Geometry: final body of the model. Coordinates: model frame, mm. A direction names the side the tool comes from. Give positions to 0.01 mm unless a question says otherwise; leave off trailing zeros. Write each loop counter-clockwise with the first axis right and the second up, starting at its lowest first coordinate (ties: lowest second). Pieces come first, ordered by that corner, then holes.
Q1. Reachability of faces 1 (the flat face through (-13, -8, 31)), 2 (the cylindrical face through (74.856, -19.944, -1.724)), 3 (the flat face through (-12, -16, 31)), 4 (the flat face through (35.699, -12, 17)) from +Z, -Z, +X, -X, +Y, -Y: full face, straight path, thin tool, end or side. Return the list, or none.
Q2. Section B-B (y = -4.75). Return the cut outline in (x, z).
Q3. Pin query (flat end, axial travel): pin 1 Ø1 at (y, z) = (-3.5, 25.5) entering from -X; pin 2 Ø1.5 at (x, y) = (53.5, -8.5) entering from +Z; pin 3 Ø2 at (x, y) = (33, -12.5) entering from +Z; pin 4 Ø14.5 at (x, z) = (46.7, 0) entering from -Y. Return the tip coordinate at first contact, or that it passes through.
Q4. Mould query, pull axis X, two halves, no side actions, for faces 5 (the flat face through (53, -8, 11)), 6 (the cylindrical face through (50.992, -19.944, 1.352)), 7 (the cylindrical face through (44.71, -17.17, 28.79)). Classes: +X half, -X half, draft (parallel to the pull), parting line (faces both ways), or undercut.
Q5. Line query: line 1 (Y direction, x = 48, z = 7); line 2 (Z direction, x = 45, y = -4.5); line 3 (X direction, y = -18.5, z = 3.5). Output: solid intervals per line, ascending.
Q6. Section A-A (x = 61.5). Return the cut outline in (y, z), plus the area to 3 significant figures.
Q7. Section D-D (y = -22). Return the cut outline in (x, z), plus the area to 3 significant figures.
Q8. Section C-C (z = 7.5). Return the cut outline in (x, y), plus the area to 3 significant figures.
from build123d import *

# Parameters (mm, degrees)
F0_R          = 4.5
F1_DEPTH      = 24
F2_W          = 44
F2_H          = 8
F3_DEPTH      = 500
F3_DEPTH_BACK = 500


with BuildPart() as f1:
    # F0 (on Front) → F1 (new body)
    with BuildSketch(Plane.XZ):
        with BuildLine():
            Line((5.0324307792, 37), (-29.3005991912, 37))
            ThreePointArc((-29.3005991912, 37), (-36.16925593, 28.6503501919), (-26.6519474056, 23.5204441728))
            ThreePointArc((-26.6519474056, 23.5204441728), (11.4307481655, 23.4196145494), (38.3961523004, -3.4721843568))
            ThreePointArc((38.3961523004, -3.4721843568), (43.8208262505, -8.5272392081), (51.1994008088, -7.7942286341))
            ThreePointArc((51.1994008088, -7.7942286341), (58.6994008088, -5.7846096908), (66.1994008088, -7.7942286341))
            ThreePointArc((66.1994008088, -7.7942286341), (77.7427343256, -5.6028075971), (77.281890635, 6.1376565306))
            ThreePointArc((77.281890635, 6.1376565306), (77.1932786056, 6.2301382417), (77.1045481967, 6.3225063811))
            ThreePointArc((77.1045481967, 6.3225063811), (44.1971429695, 29.011549922), (5.0324307792, 37))
        make_face()
        with Locations((46.6994008088, 0)):
            Circle(F0_R, mode=Mode.SUBTRACT)
        with Locations((70.6994008088, 0)):
            Circle(F0_R, mode=Mode.SUBTRACT)
    extrude(amount=F1_DEPTH)

    # F2 (on Top) → F3 (cut, two sides)
    with BuildSketch(Plane.XY) as f3_sk:
        with BuildLine():
            Line((-36.3005991912, 0), (-36.3005991912, -8))
            Line((-36.3005991912, -8), (11.2890750086, -8))
            Line((11.2890750086, -8), (14.0389679, -8))
            ThreePointArc((14.0389679, -8), (22.2442020954, -5.6035173609), (28.6994008088, 0))
            Line((28.6994008088, 0), (-36.3005991912, 0))
        make_face()
        with BuildLine():
            Line((-36.3005991912, -16), (-36.3005991912, -24))
            Line((-36.3005991912, -24), (28.6994008088, -24))
            ThreePointArc((28.6994008088, -24), (22.2442020954, -18.3964826391), (14.0389679, -16))
            Line((14.0389679, -16), (11.2890750086, -16))
            Line((11.2890750086, -16), (-36.3005991912, -16))
        make_face()
        with BuildLine():
            ThreePointArc((14.0389679, -16), (12.6640214543, -15.9526820822), (11.2890750086, -16))
            Line((11.2890750086, -16), (14.0389679, -16))
        make_face()
        with BuildLine():
            Line((14.0389679, -8), (11.2890750086, -8))
            ThreePointArc((11.2890750086, -8), (12.6640214543, -8.0473179178), (14.0389679, -8))
        make_face()
        with Locations((57.6994008088, -12)):
            Rectangle(F2_W, F2_H)
    extrude(amount=-F3_DEPTH, mode=Mode.SUBTRACT)
    extrude(f3_sk.sketch, amount=F3_DEPTH_BACK, mode=Mode.SUBTRACT)


solid = f1.part
Computed:
1. face 1: +Z, -Z, -X, +Y
1. face 2: +Y, -Y
1. face 3: +Z, -Z, -X, -Y
1. face 4: +Z, -Z, +X
2. outline: (23.66, 16.15) arc R50 cw to (38.4, -3.47) arc R9 ccw to (51.2, -7.79) arc R15 cw to (66.2, -7.79) arc R9 ccw to (77.28, 6.14) arc R100 ccw to (77.1, 6.32) arc R100 ccw to (23.66, 35.25) - close; hole circle Ø9 at (46.7, 0); hole circle Ø9 at (70.7, 0)
3. pin 1: stops at x = 24.73
3. pin 2: stops at z = 24.78
3. pin 3: stops at z = 33.3
3. pin 4: stops at y = -24
4. face 5: draft
4. face 6: undercut
4. face 7: +X half
5. line 1: y = -24 to -16, -8 to 0
5. line 2: z = -8.84 to -4.17, 4.17 to 28.67
5. line 3: x = 34.81 to 43.87, 49.53 to 67.87, 73.53 to 78.99
6. outline: (-24, -6.05) - (-16, -6.05) - (-16, 19.53) - (-24, 19.53) - close; (-8, -6.05) - (0, -6.05) - (0, 19.53) - (-8, 19.53) - close
6. area: 409 mm2
7. outline: (26.99, 13.21) arc R50 cw to (38.4, -3.47) arc R9 ccw to (51.2, -7.79) arc R15 cw to (66.2, -7.79) arc R9 ccw to (77.28, 6.14) arc R100 ccw to (77.1, 6.32) arc R100 ccw to (26.99, 34.56) - close; hole circle Ø9 at (46.7, 0); hole circle Ø9 at (70.7, 0)
7. area: 1,300 mm2
8. outline: (32.07, -24) - (75.95, -24) - (75.95, -16) - (35.7, -16) - (35.7, -8) - (75.95, -8) - (75.95, 0) - (32.07, 0) - close
8. area: 731 mm2
